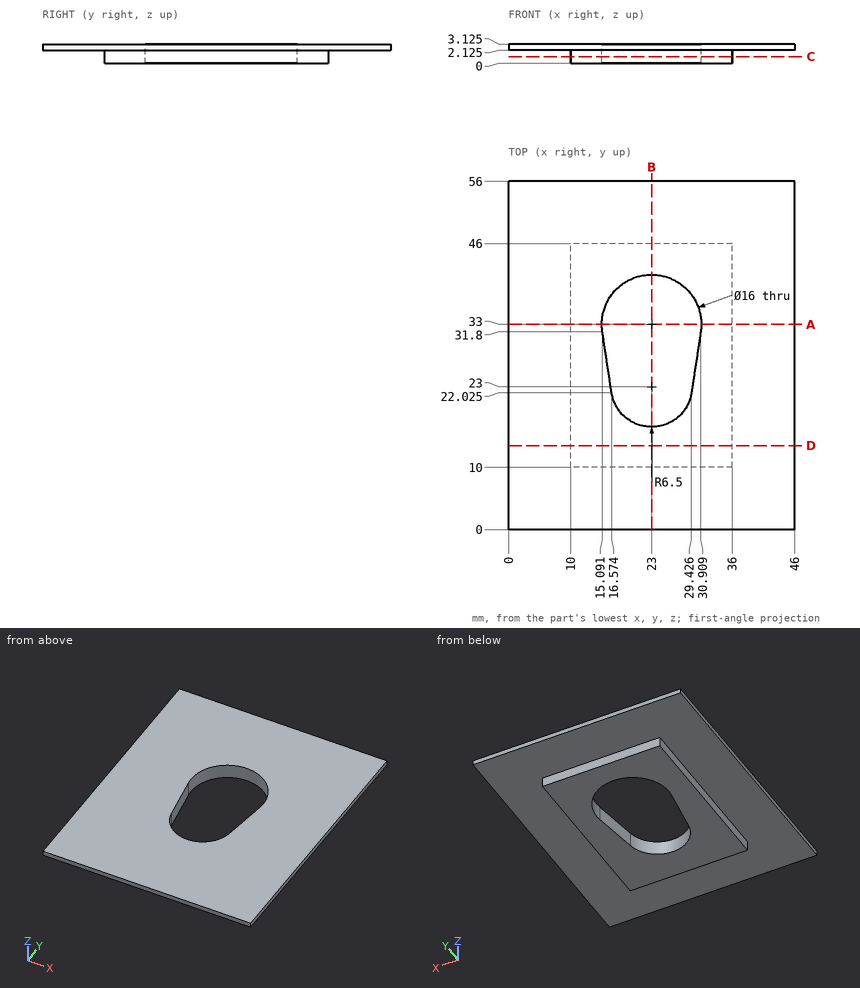
Input: dimensioned drawing with shaded views. Units: mm. Origin: part minimum x, y, z. Coordinates: 2 decimals unless noted, no trailing zeros. Loops run counter-clockwise (first coordinate to the right, second up) from the corner with the lowest first, then second, coordinate; pieces in that order, holes last. Notation, with made-up numbers: M 13.25,-4 L 54.25,-4 A33 ccw 54.25,33 Z; hole C -35,25.5 d4. An arc over 180 degrees is marked long. One line per item, written item: value. Start each with the question number.
1) Material intervals for L1, parallel to X at y = 33, z = 1.2; L2, parallel to Y at x = 23, z = 1.5; L3, parallel to Y at x = 35, z = 0.55, sorted ascending. Write a range as from..to.
2) Cut plane B-B (x = 23). Return loops of the section in (y, z) (1 decimal).
3) Cut plane A-A (y = 33). Return loops of the section in (x, z) (1 decimal).
4) Cut plane C-C (z = 1.1). Return loops of the section in (x, y) (1 decimal).
5) Pin query (flat end, axial travel): P1, Ø0.6, axis at y = 22.5, z = 1, coming from the -X side; P2, Ø1.1, axis at x = 25.5, z = 1.5, coming from the +Y side; P3, Ø0.6, axis at x = 17.5, z = 1, coming from the -Y side. Return the tip coordinate at first contact, or that it passes through.
6) Cut plane D-D (y = 13.5). Return loops of the section in (x, z) (1 decimal), then the cut area to 3 significant figures.
Evaluation:
1. L1: 10..15, 31..36
1. L2: 10..16.5, 41..46
1. L3: 10..46
2. outline: M 0,2.1 L 10,2.1 L 10,0 L 16.5,0 L 16.5,3.1 L 0,3.1 Z; M 41,0 L 46,0 L 46,2.1 L 56,2.1 L 56,3.1 L 41,3.1 Z
3. outline: M 0,2.1 L 10,2.1 L 10,0 L 15,0 L 15,3.1 L 0,3.1 Z; M 31,0 L 36,0 L 36,2.1 L 46,2.1 L 46,3.1 L 31,3.1 Z
4. outline: M 10,10 L 36,10 L 36,46 L 10,46 Z; hole M 15.1,31.8 L 16.6,22 A6.5 ccw 29.4,22 L 30.9,31.8 A8 ccw long Z
5. P1: x = 10
5. P2: y = 46
5. P3: y = 10
6. outline: M 0,2.1 L 10,2.1 L 10,0 L 36,0 L 36,2.1 L 46,2.1 L 46,3.1 L 0,3.1 Z
6. area: 101 mm^2
